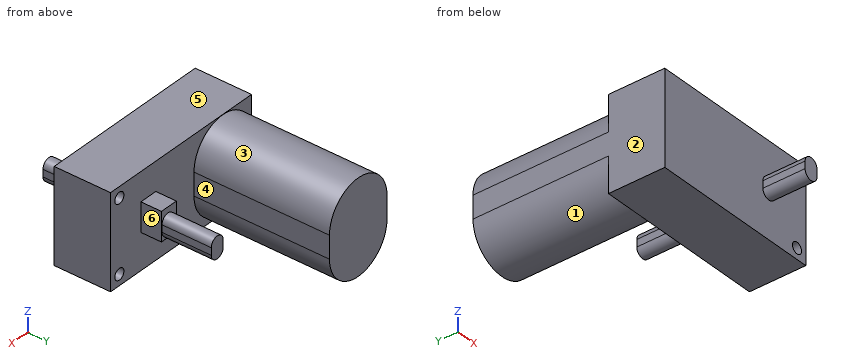
```python
from build123d import *

# Parameters (mm, degrees)
SKETCH1_W                = 42.01
SKETCH1_H                = 22.76
BOSS_EXTRUDE1_DEPTH      = 13.73
BOSS_EXTRUDE2_DEPTH      = 33
BOSS_EXTRUDE3_DEPTH      = 17
BOSS_EXTRUDE3_DEPTH_BACK = 24
SKETCH4_R                = 1.35
CUT_EXTRUDE1_DEPTH       = 17
SKETCH5_W                = 4.431132328
SKETCH5_H                = 7.028163836
BOSS_EXTRUDE4_DEPTH      = 5


with BuildPart() as part:
    # Sketch1 → Boss-Extrude1 (new body)
    with BuildSketch(Plane(origin=(0, 0, 0), x_dir=(1, 0, 0), z_dir=(0, 1, 0))):
        Rectangle(SKETCH1_W, SKETCH1_H)
    extrude(amount=BOSS_EXTRUDE1_DEPTH)

    # Sketch2 → Boss-Extrude2 (add)
    with BuildSketch(Plane(origin=(0, 13.73, 0), x_dir=(1, 0, 0), z_dir=(0, 1, 0))):
        with BuildLine():
            Line((-21.005, -2.75), (-21.005, 2.75))
            ThreePointArc((-21.005, 2.75), (-12.435, 11.32), (-3.865, 2.75))
            Line((-3.865, 2.75), (-3.865, -2.75))
            ThreePointArc((-3.865, -2.75), (-12.435, -11.32), (-21.005, -2.75))
        make_face()
    extrude(amount=BOSS_EXTRUDE2_DEPTH)

    # Sketch3 → Boss-Extrude3 (add, two sides: drawn at the far end of the back side and taken through both)
    with BuildSketch(Plane(origin=(0, 13.73, 0), x_dir=(1, 0, 0), z_dir=(0, 1, 0)).offset(-BOSS_EXTRUDE3_DEPTH_BACK)):
        with BuildLine():
            Line((8.23, -1.25), (8.23, 0.49))
            ThreePointArc((8.23, 0.49), (10.005, 2.265), (11.78, 0.49))
            Line((11.78, 0.49), (11.78, -1.25))
            ThreePointArc((11.78, -1.25), (10.005, -3.025), (8.23, -1.25))
        make_face()
    extrude(amount=BOSS_EXTRUDE3_DEPTH + BOSS_EXTRUDE3_DEPTH_BACK)

    # Sketch4 → Cut-Extrude1 (cut)
    with BuildSketch(Plane(origin=(0, 13.73, 0), x_dir=(1, 0, 0), z_dir=(0, 1, 0))):
        with Locations(Location((18.375, 8.75, 0), (0, 0, 270))):
            Circle(SKETCH4_R)
        with Locations(Location((18.375, -8.75, 0), (0, 0, 270))):
            Circle(SKETCH4_R)
    extrude(amount=-CUT_EXTRUDE1_DEPTH, mode=Mode.SUBTRACT)

    # Sketch5 → Boss-Extrude4 (add)
    with BuildSketch(Plane(origin=(0, 13.73, 0), x_dir=(1, 0, 0), z_dir=(0, 1, 0))):
        with Locations((9.740065893, -0.904904843)):
            Rectangle(SKETCH5_W, SKETCH5_H)
    extrude(amount=BOSS_EXTRUDE4_DEPTH)


solid = part.part
```
Input: part model. Units: mm. Frame: model coordinates. Face numbers are marked on the shaded views. A direction names the side the tool comes from. Give positions to 0.01 mm unless a question says otherwise; leave off trailing zeros. Write each loop counter-clockwise with the first axis right and the second up, starting at its lowest first coordinate (ties: lowest second). Pieces come first, ordered by that corner, then holes. Notation, with made-up numbers: (55.25, 7.25) - (59.25, 7.25) arc R10 ccw to (59.25, 11.25) - close; hole circle Ø10 at (-27.5, 60). An arc over 180 degrees is marked (long way). Write item = value, one per line. Start each with the question number.
1. Section query D-D, the plane x = 14. Output: boundary loops of the cut face in (y, z), then the cut area to 3 significant figures.
2. Section query C-C, the plane z = -6. Output: boundary loops of the cut face in (x, y) (3 decimals).
3. Mould query, pull axis X, two halves, no side actions, for the marked faces 4, 5 and 6. Classes: released by +X, released by -X, zero draft, split by the parting line, or undercut.
4. First-contact query: pin 1 Ø1.4 at (y, z) = (-2.5, 0.5) entering from +X; pin 2 Ø2 at (x, y) = (9, 15.5) entering from -Z; pin 3 Ø1.4 at (y, z) = (-5, 0) entering from -X. Flat tips, straight axial feed; report the tip coordinate or a pass-through.
5. Ray query, L1, parallel to X at y = 4, z = -8.75 (3 decimals); L2, parallel to Z at x = 19, y = 4; L3, parallel to Y at x = 2.5, z = 4.5. Return the intervals inside material, ascending.
6. Section query A-A, the plane y = 30. Output: boundary loops of the cut face in (x, z) (3 decimals), then the cut area to 3 significant figures.
7. Section query B-B, the plane z = -8.75. Output: boundary loops of the cut face in (x, y) (3 decimals).
8. Access query for the marked faces 1, 2 and 3. Directions: +Z, -Z, +X, -X, +Y, -Y. A direction counts if a zero-diameter tool reaches every point of the face in a straight line with its end or side. Return the directions, or none.
Check sheet entries:
q1.outline = (0, -11.38) - (13.73, -11.38) - (13.73, 11.38) - (0, 11.38) - close
q1.area = 312 mm2
q2.outline = (-21.005, 0) - (21.005, 0) - (21.005, 13.73) - (-4.505, 13.73) - (-4.505, 46.73) - (-20.365, 46.73) - (-20.365, 13.73) - (-21.005, 13.73) - close
q3.face_4 = undercut
q3.face_5 = zero draft
q3.face_6 = released by +X
q4.pin_1 = 11.78
q4.pin_2 = -2.61
q4.pin_3 = 8.23
q5.L1 = -21.005 to 17.025, 19.725 to 21.005
q5.L2 = -11.38 to -9.95, -7.55 to 7.55, 9.95 to 11.38
q5.L3 = 0 to 13.73
q6.outline = (-21.005, -2.75) arc R8.57 ccw to (-3.865, -2.75) - (-3.865, 2.75) arc R8.57 ccw to (-21.005, 2.75) - close; (8.23, -0.49) arc R1.775 ccw to (11.78, -0.49) - (11.78, 1.25) arc R1.775 ccw to (8.23, 1.25) - close
q6.area = 341 mm2
q7.outline = (-21.005, 0) - (17.025, 0) - (17.025, 13.73) - (-6.316, 13.73) - (-6.316, 46.73) - (-18.554, 46.73) - (-18.554, 13.73) - (-21.005, 13.73) - close; (19.725, 0) - (21.005, 0) - (21.005, 13.73) - (19.725, 13.73) - close
q8.face_1 = -Z, +Y
q8.face_2 = +Z, -Z, -X, +Y, -Y
q8.face_3 = +Z, +Y
